Check sheet for the drawn part. Datum: minimum x, y, z corner. Units: mm. A direction names the side the tool comes from. Round coordinates to 2 decimals unless told otherwise and drop trailing zeros. Write each loop counter-clockwise with the first axis right and the second up, starting at its lowest first coordinate (ties: lowest second). Pieces come first, ordered by that corner, then holes. Notation, with made-up numbers: (84.25, 31) - (131.25, 31) arc R12 cw to (131.25, 53) - close; hole circle Ø10 at (-36, 68). An arc over 180 degrees is marked (long way). Answer as a JSON object with one key per item and string values.
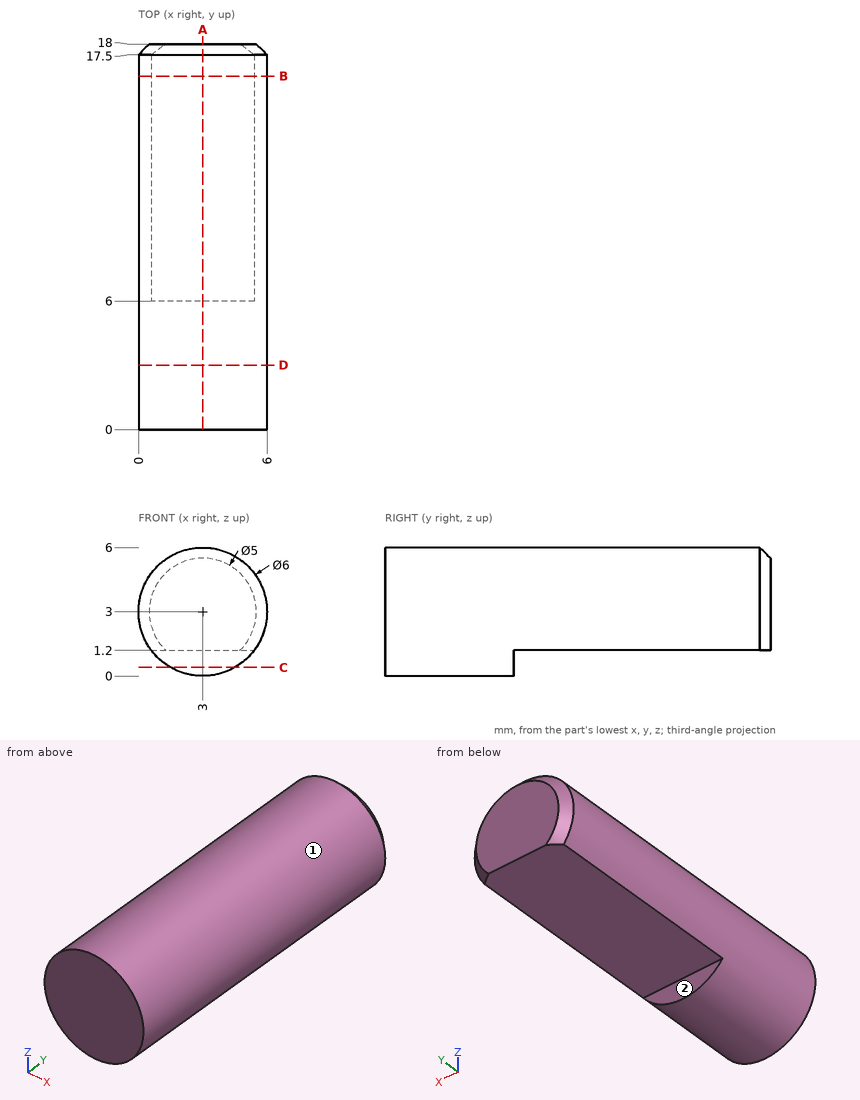
1. Go/stop test with flat-tipped pins: pin 1 (1 mm diameter, centred on x = 4, z = 0.5, fed in from +Y); pin 2 (3 mm diameter, centred on x = 4.5, z = 1.5, fed in from -Y). Record where each tip stops, or that it passes through.
Completed:
{"pin 1": "stops at y = 6", "pin 2": "stops at y = 0"}
2. Material ranges on probe 1 along X at (y, z) = (2.5, 4.8); probe 2 along X at (y, z) = (9.25, 5.7); probe 3 along Z at (x, y) = (4.7, 9.75), recorded low to high. Write a range as from..to.
Completed:
{"probe 1": "x = 0.6..5.4", "probe 2": "x = 1.69..4.31", "probe 3": "z = 1.2..5.47"}
3. Cross-section at B-B (y = 16.5). Record the boundary of the cut face in (x, z).
Completed:
{"outline": "(0.6, 1.2) - (5.4, 1.2) arc R3 ccw (long way) to start"}
4. Access from +Z, -Z, +X, -X, +Y, -Y to the whole of each face (thin tool, end or side, straight path). Record for the marked faces 1 and 2.
Completed:
{"face 1": "+Y, -Y", "face 2": "-Z, +X, -X, +Y"}
5. Cross-section at C-C (z = 0.4). Record the boundary of the cut face in (x, y), plus the area to 3 significant figures.
Completed:
{"outline": "(1.5, 0) - (4.5, 0) - (4.5, 6) - (1.5, 6) - close", "area": "18.0 mm^2"}
6. Cross-section at A-A (x = 3). Record the boundary of the cut face in (y, z), plus the area to 3 significant figures.
Completed:
{"outline": "(0, 0) - (6, 0) - (6, 1.2) - (18, 1.2) - (18, 5.5) - (17.5, 6) - (0, 6) - close", "area": "93.5 mm^2"}
7. Cross-section at D-D (y = 3). Record the boundary of the cut face in (x, z).
Completed:
{"outline": "circle Ø6 at (3, 3)"}
